```python
from build123d import *

# Parameters (mm, degrees)
F1_DEPTH = 19.05
F2_W     = 25.4
F2_H     = 66.675
F3_DEPTH = 25.4
F5_DEPTH = 32.258


with BuildPart() as f1:
    # F0 (on Top) → F1 (new body)
    with BuildSketch(Plane.XY):
        Polygon((53.38208, 34.755277), (-31.990739, 34.755277), (-31.990739, -31.919723), (54.581683, -31.919723), (88.659261, -12.245024), (88.659261, -6.519723), (31.509261, -6.519723), (31.509261, 9.355277), (88.659261, 9.355277), (88.659261, 14.387987), align=None)
    extrude(amount=F1_DEPTH)

    # F2 (on face) → F3 (join)
    with BuildSketch(Plane.XY.offset(19.05)):
        with Locations((-19.290739, 1.417777)):
            Rectangle(F2_W, F2_H)
    extrude(amount=F3_DEPTH)

    # F4 (on face) → F5 (cut)
    with BuildSketch(Plane.YZ.offset(-6.590739)):
        Polygon((15.705277, 44.45), (-12.869723, 44.45), (-19.578354, 32.83031), (22.413908, 32.83031), align=None)
    extrude(amount=-F5_DEPTH, mode=Mode.SUBTRACT)


solid = f1.part
```
Can you work these out from the model? Positions are in its coordinate system, mm. A direction names the side the tool comes from. Round coordinates to 2 decimals unless told otherwise and drop trailing zeros. Loops run counter-clockwise (first coordinate to the right, second up) from the corner with the lowest first, then second, coordinate; pieces in that order, holes last. Notation, with made-up numbers: M -16,53.25 L -10,53.25 A34 ccw -10,92.25 Z; hole C -14,78.25 d2. An arc over 180 degrees is marked long. Answer as a JSON object with one key per item and string values. Group by question number.
Q1. On a 3-axis mill with a long thin cutter (end or side, diameter ignored), from which of +Z, -Z, +X, -X, +Y, -Y can I reach the whole of each face in a straight line? I mean faces 1 (the flat face through (31.509, 1, 9)), 2 (the flat face through (-19, 1, 32.83)), 3 (the flat face through (-6.591, 1, 29)). Say none if no direction works.
Q2. Will these pins go through, and if not, where does the flat tip stop? pin 1 (6 mm diameter, centred on x = 72.5, y = -25, fed in from +Z); pin 2 (21 mm diameter, centred on x = 68.5, z = 8, fed in from -Y); pin 3 (7.5 mm diameter, centred on x = -15, y = 7.5, fed in from +Z); pin 4 (10 mm diameter, centred on y = 17, z = 33, fed in from -X).
Q3. Imagine slicing it at A-A, the plane x = 46. Please give me the cut outline in (y, z).
Q4. Imagine slicing it at D-D, the plane x = -10. Please give me the cut outline in (y, z), then the cut area to 3 significant figures.
Q5. Imagine slicing it at C-C, the plane y = -18. Please give me the cut outline in (x, z).
Q6. Please list where these lines run through material, in increasing order: L1, parallel to Y at x = 48, z = 17; L2, parallel to Z at x = 50, y = -9; L3, parallel to Y at x = -19, z = 34.
Q7. Imagine slicing it at B-B, the plane z = 35. Please give me the cut outline in (x, y).
Findings:
{
 "1": {"face 1": "+Z, -Z, +X", "face 2": "+X, -X", "face 3": "+Z, +X, +Y, -Y"},
 "2": {"pin 1": "stops at z = 19.05", "pin 2": "stops at y = -29.95", "pin 3": "stops at z = 32.83", "pin 4": "stops at x = -31.99"},
 "3": {"outline": "M -31.92,0 L -6.52,0 L -6.52,19.05 L -31.92,19.05 Z; M 9.36,0 L 34.76,0 L 34.76,19.05 L 9.36,19.05 Z"},
 "4": {"outline": "M -31.92,0 L 34.76,0 L 34.76,44.45 L 15.71,44.45 L 22.41,32.83 L -19.58,32.83 L -12.87,44.45 L -31.92,44.45 Z", "area": "2,550 mm2"},
 "5": {"outline": "M -31.99,0 L 78.69,0 L 78.69,19.05 L -6.59,19.05 L -6.59,32.83 L -31.99,32.83 Z; M -31.99,35.56 L -6.59,35.56 L -6.59,44.45 L -31.99,44.45 Z"},
 "6": {"L1": "y = -31.92 to -6.52, 9.36 to 34.76", "L2": "z = 0 to 19.05", "L3": "y = -31.92 to -18.9, 21.74 to 34.76"},
 "7": {"outline": "M -31.99,-31.92 L -6.59,-31.92 L -6.59,-18.33 L -31.99,-18.33 Z; M -31.99,21.16 L -6.59,21.16 L -6.59,34.76 L -31.99,34.76 Z"}
}
